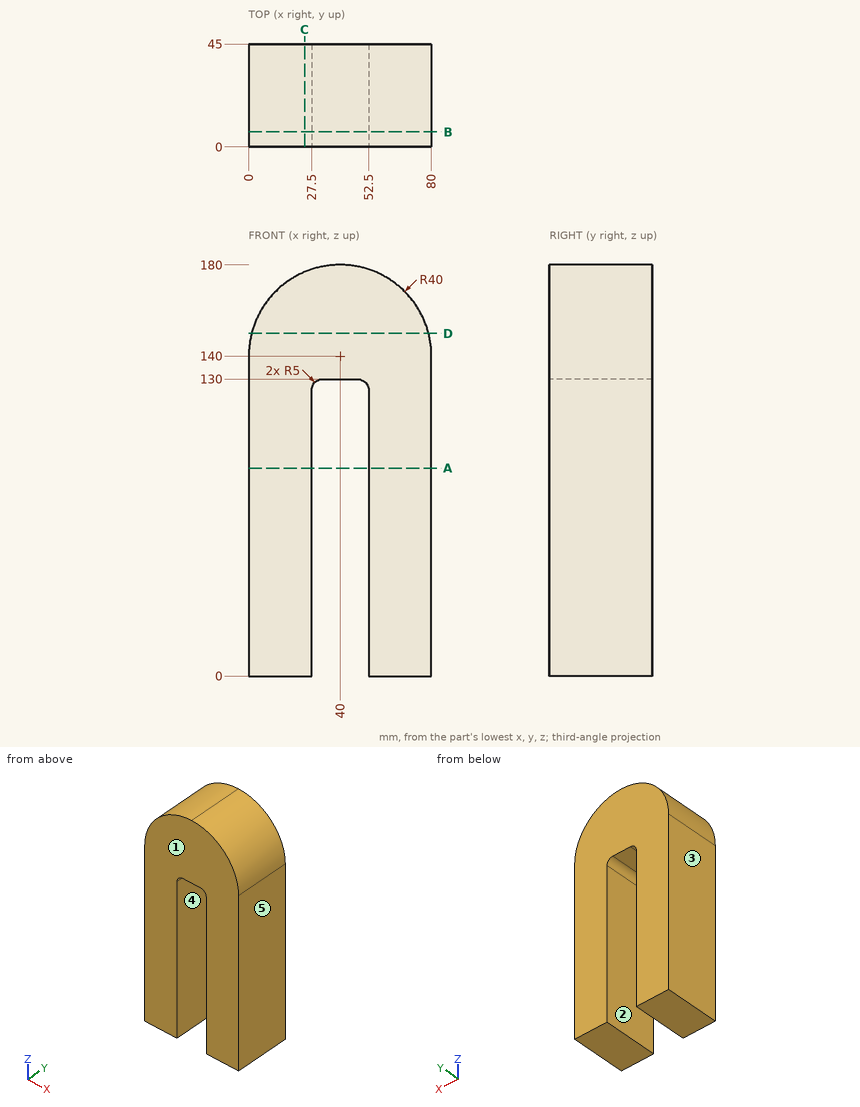
Source: three-view drawing plus pictorial views. Frame: mm from the lowest corner of the part. A direction names the side the tool comes from. Give positions to 0.01 mm unless a question says otherwise; leave off trailing zeros. Write each loop counter-clockwise with the first axis right and the second up, starting at its lowest first coordinate (ties: lowest second). Pieces come first, ordered by that corner, then holes. Notation, with made-up numbers: (86.25, 40) - (90.25, 40) arc R5 ccw to (90.25, 47) - close; hole circle Ø4 at (-10, 27.5). An arc over 180 degrees is marked (long way). Write item = value, one per line. Start each with the question number.
1. First-contact query: pin 1 Ø8 at (x, y) = (27.5, 14.5) entering from +Z; pin 2 Ø7.5 at (x, y) = (40, 11.5) entering from -Z. Flat tips, straight axial feed; report the tip coordinate or a pass-through.
2. Section query D-D, the plane z = 150. Output: boundary loops of the cut face in (x, y).
3. Section query C-C, the plane x = 24.5. Output: boundary loops of the cut face in (y, z), then the cut area to 3 significant figures.
4. Mould query, pull axis X, two halves, no side actions, for the marked faces 1, 2 and 3. Classes: released by +X, released by -X, zero draft, split by the parting line, or undercut.
5. Ray query, L1, parallel to X at y = 23.5, z = 80; L2, parallel to X at y = 36.5, z = 146.5; L3, parallel to Z at x = 9.5, y = 33.5. Return the intervals inside material, ascending.
6. Access query for the marked faces 4 and 5. Directions: +Z, -Z, +X, -X, +Y, -Y. A direction counts if a zero-diameter tool reaches every point of the face in a straight line with its end or side. Return the directions, or none.
7. Section query A-A, the plane z = 91. Output: boundary loops of the cut face in (x, y).
8. Section query B-B, the plane y = 6.5. Output: boundary loops of the cut face in (x, z).
Check sheet entries:
q1.pin_1 = 179.09
q1.pin_2 = 130
q2.outline = (1.27, 0) - (78.73, 0) - (78.73, 45) - (1.27, 45) - close
q3.outline = (0, 0) - (45, 0) - (45, 176.87) - (0, 176.87) - close
q3.area = 7,960 mm2
q4.face_1 = zero draft
q4.face_2 = undercut
q4.face_3 = released by -X
q5.L1 = 0 to 27.5, 52.5 to 80
q5.L2 = 0.53 to 79.47
q5.L3 = 0 to 165.88
q6.face_4 = -Z, +Y, -Y
q6.face_5 = +Z, -Z, +X, +Y, -Y
q7.outline = (0, 0) - (27.5, 0) - (27.5, 45) - (0, 45) - close; (52.5, 0) - (80, 0) - (80, 45) - (52.5, 45) - close
q8.outline = (0, 0) - (27.5, 0) - (27.5, 125) arc R5 cw to (32.5, 130) - (47.5, 130) arc R5 cw to (52.5, 125) - (52.5, 0) - (80, 0) - (80, 140) arc R40 ccw to (40, 180) arc R40 ccw to (0, 140) - close
